Part print with two shaded views. Sizes in mm from the minimum x, y, z corner. Give positions to 0.01 mm unless a question says otherwise; leave off trailing zeros. Write each loop counter-clockwise with the first axis right and the second up, starting at its lowest first coordinate (ties: lowest second). Pieces come first, ordered by that corner, then holes. Notation, with made-up numbers: (-15.75, -26) - (-2.75, -26) arc R16 ccw to (-2.75, -22) - close; hole circle Ø4 at (-32, 68). An arc over 180 degrees is marked (long way). Answer as a JSON object with one key per item and string values.
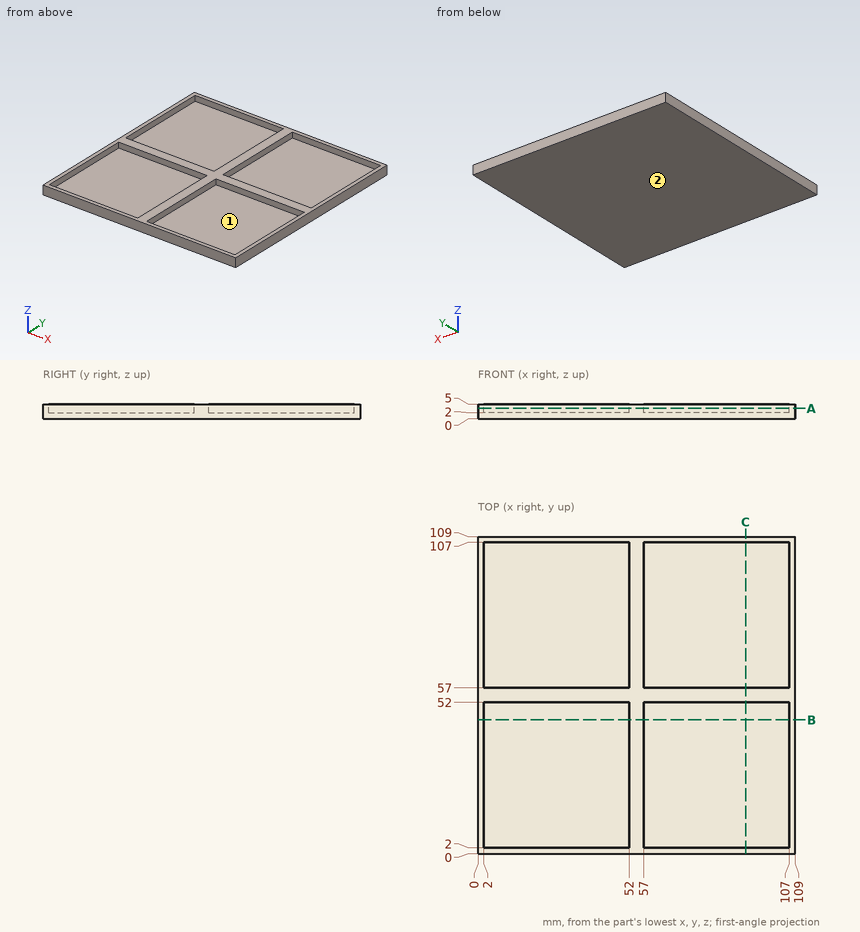
(1) Flat gauge pin, fed straight in: P1, Ø10, axis at x = 26, y = 71.5, coming from the +Z side. Where does the tip first touch, or does it go through?
Answer key:
{"P1": "stops at z = 2"}
(2) Saw through at A-A, the plane z = 3.5. Give the cut face in (x, y).
Answer key:
{"outline": "(0, 0) - (109, 0) - (109, 109) - (0, 109) - close; hole (2, 2) - (52, 2) - (52, 52) - (2, 52) - close; hole (2, 57) - (52, 57) - (52, 107) - (2, 107) - close; hole (57, 2) - (107, 2) - (107, 52) - (57, 52) - close; hole (57, 57) - (107, 57) - (107, 107) - (57, 107) - close"}
(3) Pull direction X, two halves, no side cores. Call the marked faces 1 and 2: pulls with the +X half, pulls with the -X half, needs draft (parallel to the pull), parting line crosses it, or undercut.
Answer key:
{"face 1": "undercut", "face 2": "needs draft"}
(4) Probe L1, parallel to Y at x = 23.5, z = 3.85; L2, parallel to Z at x = 42, y = 36.5. List the from-to ranges inside material, lowest first. Write a range as [from, to].
Answer key:
{"L1": "y = [0, 2], [52, 57], [107, 109]", "L2": "z = [0, 2]"}
(5) Saw through at B-B, the plane y = 46. Give the cut face in (x, z), and give its area (3 significant figures).
Answer key:
{"outline": "(0, 0) - (109, 0) - (109, 5) - (107, 5) - (107, 2) - (57, 2) - (57, 5) - (52, 5) - (52, 2) - (2, 2) - (2, 5) - (0, 5) - close", "area": "245 mm²"}
